Geometry check sheet. Reference: the model listing, model coordinates, mm. Give positions to 0.01 mm unless a question says otherwise; leave off trailing zeros. Loops run counter-clockwise (first coordinate to the right, second up) from the corner with the lowest first, then second, coordinate; pieces in that order, holes last. Notation, with made-up numbers: (-11, 47) -> (33, 47) arc R20 cw to (33, 61) -> close; hole circle Ø1 at (-34, 33.5). An arc over 180 degrees is marked (long way). One line per question, with ' | ' between items.
Autodesk Inventor part; units mm, degrees
ref_plane "YZ Plane" through (0, 0, 0) normal (1, 0, 0) x (0, 1, 0)
ref_plane "XZ Plane" through (0, 0, 0) normal (0, 1, 0) x (-1, 0, 0)
ref_plane "XY Plane" through (0, 0, 0) normal (0, 0, 1) x (1, 0, 0)
sketch "Sketch1" plane through (0, 0, 0) normal (0, 0, 1) x (1, 0, 0)
  line L0 (0, 0) -> (10, 0)
  line L1 (10, 0) -> (10, 25)
  line L2 (10, 25) -> (0, 25)
  line L3 (0, 25) -> (0, 0)
  dimension "d0" = 10
  dimension "d1" = 25
extrude "Extrusion1" add sketch "Sketch1" along normal blind 6
sketch "Sketch2" plane through (0, 0, 6) normal (0, 0, 1) x (1, 0, 0)
  line L0 (10, 0) -> (10, 25) construction
  line L1 (10, 25) -> (0, 25) construction
  line L2 (0, 25) -> (0, 0) construction
  line L3 (0, 0) -> (10, 0) construction
  point P0 (5, 20)
  point P1 (5, 5)
  dimension "d4" = 5
  dimension "d5" = 10
  dimension "d6" = 5
  dimension "d7" = 5
  dimension "d15" = 15
hole "Hole1" at (5, 20, 6) at (5, 5, 6) direction (0, 0, -1) diameter 3.242 end through all
properties part number "Flange attach block"
Item 1: Sectioned sample at B-B (x = 5). Record the cut outline in (y, z).
Result:
outline: (0, 0) -> (3.38, 0) -> (3.38, 6) -> (0, 6) -> close; (6.62, 0) -> (18.38, 0) -> (18.38, 6) -> (6.62, 6) -> close; (21.62, 0) -> (25, 0) -> (25, 6) -> (21.62, 6) -> close
Item 2: Sectioned sample at D-D (y = 19.5). Record the cut outline in (x, z).
Result:
outline: (0, 0) -> (3.46, 0) -> (3.46, 6) -> (0, 6) -> close; (6.54, 0) -> (10, 0) -> (10, 6) -> (6.54, 6) -> close
Item 3: Sectioned sample at A-A (y = 5). Record the cut outline in (x, z).
Result:
outline: (0, 0) -> (3.38, 0) -> (3.38, 6) -> (0, 6) -> close; (6.62, 0) -> (10, 0) -> (10, 6) -> (6.62, 6) -> close
Item 4: Release check for a two-part mould opening along Y. For faces 1 (the face through (10, 12, 3)), 2 (the face through (5, 25, 3)), 3 (the face through (5.986, 6.286, 2.958)), 4 (the face through (4.513, 18.454, 2.958)) record: pulls with the +Y half, pulls with the -Y half, needs draft (parallel to the pull), parting line crosses it, or undercut.
Result:
face 1: needs draft | face 2: pulls with the +Y half | face 3: undercut | face 4: undercut
Item 5: Scan lines: probe 1 along Y at (x, z) = (5, 3.5); probe 2 along X at (y, z) = (20, 3.8); probe 3 along Y at (x, z) = (6.25, 4.5). Record each from-to range of solid material in increasing order.
Result:
probe 1: 0 to 3.38, 6.62 to 18.38, 21.62 to 25 | probe 2: 0 to 3.38, 6.62 to 10 | probe 3: 0 to 3.97, 6.03 to 18.97, 21.03 to 25
Item 6: Sectioned sample at C-C (z = 5.35). Record the cut outline in (x, y).
Result:
outline: (0, 0) -> (10, 0) -> (10, 25) -> (0, 25) -> close; hole circle Ø3.24 at (5, 5); hole circle Ø3.24 at (5, 20)
